Design review of the part built by this model. Coordinates are the model's own, in mm. A direction names the side the tool comes from. Coordinates: 2 decimals unless noted, no trailing zeros. Write each loop counter-clockwise with the first axis right and the second up, starting at its lowest first coordinate (ties: lowest second). Pieces come first, ordered by that corner, then holes. Notation, with made-up numbers: (38.5, 48.25) - (55.5, 48.25) arc R22 cw to (55.5, 82.25) - close; hole circle Ø7 at (-2, 51). An arc over 180 degrees is marked (long way). Answer as a JSON object with one key per item and string values.
Autodesk Inventor part; units mm, degrees
ref_plane "YZ Plane" through (0, 0, 0) normal (1, 0, 0) x (0, 1, 0)
ref_plane "XZ Plane" through (0, 0, 0) normal (0, 1, 0) x (-1, 0, 0)
ref_plane "XY Plane" through (0, 0, 0) normal (0, 0, 1) x (1, 0, 0)
sketch "草圖1" plane through (0, 0, 0) normal (1, 0, 0) x (0, 1, 0)
  line L0 (0, 0) -> (45, 0)
  line L1 (45, 0) -> (45, -42)
  line L2 (45, -42) -> (85, -42)
  line L3 (85, -42) -> (85, -60)
  line L4 (85, -60) -> (0, -60)
  line L5 (0, -60) -> (0, 0)
  dimension "d0" = 60
  dimension "d1" = 85
  dimension "d2" = 42
  dimension "d3" = 40
revolve "迴轉1" add sketch "草圖1" angle 360 about axis through (0, 0, -60) along (0, 0, 1)
sketch "草圖2" plane through (0, 0, -42) normal (0, 0, 1) x (1, 0, 0)
  circle A0 centre (0, 0) radius 70 construction
  circle A1 centre (0, 70) radius 8
  circle A2 centre (-49.4975, 49.4975) radius 8
  circle A3 centre (-70, 0) radius 8
  circle A4 centre (-49.4975, -49.4975) radius 8
  circle A5 centre (0, -70) radius 8
  circle A6 centre (49.4975, -49.4975) radius 8
  circle A7 centre (70, 0) radius 8
  circle A8 centre (49.4975, 49.4975) radius 8
  dimension "d5" = 140
  dimension "d6" = 16
  dimension "d7" = 70
  dimension "d12" = 360
extrude "擠出1" cut sketch "草圖2" against normal up to next
sketch "草圖4" plane through (0, 0, 0) normal (0, 0, 1) x (1, 0, 0)
  circle A0 centre (0, 0) radius 35
  dimension "d14" = 70
extrude "擠出2" cut sketch "草圖4" against normal up to next
fillet "圓角1" radius 5 2 edges at (0, -45, -42) (0, -85, -42)
properties part number "410571040-T3"
(1) Take a section at D-D, the plane z = -17. Write out the cut boundary in (x, y).
Solved:
{"outline": "circle Ø90 at (0, 0); hole circle Ø70 at (0, 0)"}
(2) Take a section at A-A, the plane x = 0. Write out the cut boundary in (y, z).
Solved:
{"outline": "(-85, -60) - (-78, -60) - (-78, -42) - (-80, -42) arc R5 ccw to (-85, -47) - close; (-62, -60) - (-35, -60) - (-35, 0) - (-45, 0) - (-45, -37) arc R5 cw to (-50, -42) - (-62, -42) - close; (35, -60) - (62, -60) - (62, -42) - (50, -42) arc R5 cw to (45, -37) - (45, 0) - (35, 0) - close; (78, -60) - (85, -60) - (85, -47) arc R5 ccw to (80, -42) - (78, -42) - close"}
(3) The part is to be moulded in two halves that separate along X. For faces 1 (the face through (-1, 37, -60)), 2 (the face through (-1.041, 77.932, -50.874)), 3 (the face through (-51.721, -67.453, -53.591)), say which applies: pulls with the +X half, pulls with the -X half, needs draft (parallel to the pull), parting line crosses it, or undercut.
Solved:
{"face 1": "needs draft", "face 2": "undercut", "face 3": "parting line crosses it"}
(4) To check wall thickness, follow line 1 (X direction, y = 49, z = -47); line 2 (Y direction, x = 0, z = -34); line 3 (Y direction, x = -4.5, z = -46). State the ranges of each line that lie inside material, in increasing order. Write a range as from..to.
Solved:
{"line 1": "x = -69.46..-57.48, -41.51..41.51, 57.48..69.46", "line 2": "y = -45..-35, 35..45", "line 3": "y = -84.78..-76.61, -63.39..-34.71, 34.71..63.39, 76.61..84.78"}
(5) Tool access review of faces 4 (the face through (-1.041, -62.068, -50.874)), 5 (the face through (-1, 52, -42)): name each direction out of +Z, -Z, +X, -X, +Y, -Y from which nothing blocks a thin tool from reaching the whole face with its end or side.
Solved:
{"face 4": "+Z, -Z", "face 5": "+Z"}
(6) Take a section at C-C, the plane z = -53.5. Give the number of separate pieces and of enclosed holes in the cut face, and give its area (3 significant figures).
Solved:
{"separate pieces": "1", "enclosed holes": "9", "area": "17,200 mm^2"}
(7) For pin 1 (3 mm diameter, centred on y = 31, z = -12, fed in from +X); pin 2 (2 mm diameter, centred on x = -18.5, z = -34, fed in from -Y); pin 3 (1.5 mm diameter, centred on y = -24, z = -14, fed in from +X), all flat-tipped, find the tip position at first contact; note any pin that passes through.
Solved:
{"pin 1": "stops at x = 33.98", "pin 2": "stops at y = -41.46", "pin 3": "stops at x = 38.53"}
